Read the model definition and answer for the solid it produces. Units are mm, in the model's axes. Face numbers are marked on the shaded views. A direction names the side the tool comes from. Round coordinates to 2 decimals unless told otherwise and drop trailing zeros. Order: outer loops, then holes, each group sorted by start corner. A loop starts at its lowest first (then second) coordinate and runs counter-clockwise, first axis right, second up. Notation, with made-up numbers: (-22.5, -4) -> (33.5, -4) arc R31 ccw to (33.5, 21) -> close; hole circle Ø2 at (80, -27). An arc over 180 degrees is marked (long way). One line per item, written item: value. Start each with the question number.
1. Consider line 1 (Y direction, x = 0, z = 5.25); line 2 (Z direction, x = 2.5, y = -2); line 3 (Z direction, x = 3, y = -2.75). Determine where each line is inside the solid, lowest interval first.
2. For the marked faces 1 and 2, determine the directions among +Z, -Z, +X, -X, +Y, -Y from which every point of the face is accessible in a straight line to the end or side of a thin tool.
3. Section C-C (y = 0) is taken. Give the vertices of the cut face in (x, z).
4. Section D-D (z = 7.25) is taken. Give the vertices of the cut face in (x, y), then the cut area to 3 significant figures.
5. Flat-ended cylindrical pins translate along their axes: pin 1 Ø0.5 at (x, z) = (0.5, 20.5) entering from +Y; pin 2 Ø1.2 at (y, z) = (2, 23.5) entering from +X; pin 3 Ø6 at (y, z) = (3.5, 22) entering from -X. Find the tip coordinate at first contact, or state that the pin passes through.
6. Section B-B (x = 0) is taken. Give the vertices of the cut face in (y, z), then the cut area to 3 significant figures.
7. Section A-A (z = 19) is taken. Give the vertices of the cut face in (x, y), then the cut area to 4 significant figures.
from build123d import *

# Parameters (mm, degrees)
CYLINDER002_R     = 4
CYLINDER002_DEPTH = 2
CYLINDER001_R     = 1.55
CYLINDER001_DEPTH = 9
BOX_W             = 10
BOX_H             = 2.5
BOX_DEPTH         = 11
CYLINDER_R        = 8
CYLINDER_DEPTH    = 11
FILLET002_R       = 3
BOX002_W          = 4.6
BOX002_H          = 1.7
BOX002_DEPTH      = 15
FILLET001_R       = 1
BOX001_W          = 1.7
BOX001_H          = 4.6
BOX001_DEPTH      = 15
FILLET_R          = 1


with BuildPart() as cilindro002:
    # Cylinder002 → Cylinder002 (new body)
    with BuildSketch(Plane.XY.offset(11)):
        Circle(CYLINDER002_R)
    extrude(amount=CYLINDER002_DEPTH)


with BuildPart() as cilindro001:
    # Cylinder001 → Cylinder001 (new body)
    with BuildSketch(Plane.XY):
        Circle(CYLINDER001_R)
    extrude(amount=CYLINDER001_DEPTH)


with BuildPart() as taladro:
    # Box → Box (new body)
    with BuildSketch(Plane(origin=(-5, -1.55, 0), x_dir=(1, 0, 0), z_dir=(0, 0, 1))):
        with Locations((5, 1.25)):
            Rectangle(BOX_W, BOX_H)
    extrude(amount=BOX_DEPTH)

    # Common: intersect Cilindro001
    add(cilindro001.part, mode=Mode.INTERSECT)


with BuildPart() as fillet002:
    # Cylinder → Cylinder (new body)
    with BuildSketch(Plane.XY):
        Circle(CYLINDER_R)
    extrude(amount=CYLINDER_DEPTH)

    # Cut: cut Taladro
    add(taladro.part, mode=Mode.SUBTRACT)

    # Fillet002
    fillet002_edges = [fillet002.edges().sort_by_distance(p)[0] for p in [
        (-8, 0, 11),
    ]]
    fillet(fillet002_edges, radius=FILLET002_R)


with BuildPart() as fillet001:
    # Box002 → Box002 (new body)
    with BuildSketch(Plane(origin=(-2.3, -0.85, 22), x_dir=(1, 0, 0), z_dir=(0, 0, 1))):
        with Locations((2.3, 0.85)):
            Rectangle(BOX002_W, BOX002_H)
    extrude(amount=BOX002_DEPTH)

    # Fillet001
    fillet001_edges = [fillet001.edges().sort_by_distance(p)[0] for p in [
        (-2.3, 0, 37),
        (2.3, 0, 37),
    ]]
    fillet(fillet001_edges, radius=FILLET001_R)


with BuildPart() as eje_rueda_motor:
    # Box001 → Box001 (new body)
    with BuildSketch(Plane(origin=(-0.85, -2.3, 22), x_dir=(1, 0, 0), z_dir=(0, 0, 1))):
        with Locations((0.85, 2.3)):
            Rectangle(BOX001_W, BOX001_H)
    extrude(amount=BOX001_DEPTH)

    # Fillet
    fillet_edges = [eje_rueda_motor.edges().sort_by_distance(p)[0] for p in [
        (0, -2.3, 37),
        (0, 2.3, 37),
    ]]
    fillet(fillet_edges, radius=FILLET_R)

    # Fusion: union Fillet001
    add(fillet001.part)


with BuildPart() as eje_rueda_motor_1:
    # Fusion placement: moved
    add(eje_rueda_motor.part.moved(Location((0, 0, -9))))

    # Fusion001: union Cilindro002, Fillet002
    add(cilindro002.part)
    add(fillet002.part)


solid = eje_rueda_motor_1.part
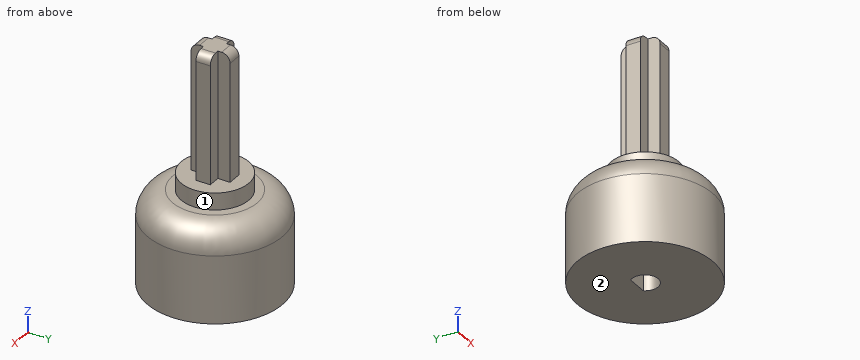
Answer:
1. line 1: -8 to -1.55, 0.95 to 8
1. line 2: 0 to 13
1. line 3: 0 to 11
2. face 1: +Z
2. face 2: -Z, +X, -X, +Y, -Y
3. outline: (-8, 0) -> (-1.55, 0) -> (-1.55, 9) -> (1.55, 9) -> (1.55, 0) -> (8, 0) -> (8, 8) arc R3 ccw to (5, 11) -> (4, 11) -> (4, 13) -> (2.3, 13) -> (2.3, 27) arc R1 ccw to (1.3, 28) -> (-1.3, 28) arc R1 ccw to (-2.3, 27) -> (-2.3, 13) -> (-4, 13) -> (-4, 11) -> (-5, 11) arc R3 ccw to (-8, 8) -> close
4. outline: circle Ø16 at (0, 0); hole (-1.22, 0.95) arc R1.55 ccw (long way) to (1.22, 0.95) -> close
4. area: 195 mm^2
5. pin 1: y = 2.3
5. pin 2: x = 0.85
5. pin 3: x = -2.3
6. outline: (-8, 0) -> (-1.55, 0) -> (-1.55, 9) -> (0.95, 9) -> (0.95, 0) -> (8, 0) -> (8, 8) arc R3 ccw to (5, 11) -> (4, 11) -> (4, 13) -> (2.3, 13) -> (2.3, 27) arc R1 ccw to (1.3, 28) -> (-1.3, 28) arc R1 ccw to (-2.3, 27) -> (-2.3, 13) -> (-4, 13) -> (-4, 11) -> (-5, 11) arc R3 ccw to (-8, 8) -> close
6. area: 234 mm^2
7. outline: (-2.3, -0.85) -> (-0.85, -0.85) -> (-0.85, -2.3) -> (0.85, -2.3) -> (0.85, -0.85) -> (2.3, -0.85) -> (2.3, 0.85) -> (0.85, 0.85) -> (0.85, 2.3) -> (-0.85, 2.3) -> (-0.85, 0.85) -> (-2.3, 0.85) -> close
7. area: 12.75 mm^2
